```python
from build123d import *

# Parameters (mm, degrees)
F1_DEPTH  = 25.4
F2_R      = 6.2861798015
F2_R_2    = 6.4106702401
F3_DEPTH  = 12.8915009478
F5_DEPTH  = 12.8915009478
F7_DEPTH  = 69.5320936104
F10_DEPTH = 9.335500879


with BuildPart() as f1:
    # F0 (on Front) → F1 (new body)
    with BuildSketch(Plane.XZ):
        Polygon((0, 31.9150984287), (0, 0), (69.6087032557, 0), (69.6087032557, 12.8905009478), (9.334500879, 12.8905009478), (9.334500879, 31.9150984287), align=None)
    extrude(amount=F1_DEPTH)

    # F2 (on face) → F3 (cut, through all)
    with BuildSketch(Plane.XY.offset(12.8905009478)):
        with Locations((48.8061010838, -12.3570999131)):
            Circle(F2_R)
        with Locations((24.6252994984, -12.7127002925)):
            Circle(F2_R_2)
    extrude(amount=-F3_DEPTH, mode=Mode.SUBTRACT)

    # F4 (on face) → F5 (cut, through all)
    with BuildSketch(Plane.XY.offset(12.8905009478)):
        with BuildLine():
            ThreePointArc((60.931898555, 0), (69.4846296944, -13.5080407898), (58.7982981412, -25.4))
            Line((58.7982981412, -25.4), (69.6087032557, -25.4))
            Line((69.6087032557, -25.4), (69.6087032557, 0))
            Line((69.6087032557, 0), (60.931898555, 0))
        make_face()
    extrude(amount=-F5_DEPTH, mode=Mode.SUBTRACT)

    # F6 (on face) → F7 (cut, through all)
    with BuildSketch(Plane(origin=(0, 0, 0), x_dir=(0, -1, 0), z_dir=(-1, 0, 0))):
        with BuildLine():
            ThreePointArc((0, 21.0692994297), (3.4400048541, 28.1838195258), (10.4061793669, 31.9150984287))
            Line((10.4061793669, 31.9150984287), (0, 31.9150984287))
            Line((0, 31.9150984287), (0, 21.0692994297))
        make_face()
        with BuildLine():
            ThreePointArc((14.9166792368, 31.9150984287), (22.126877753, 27.9222549677), (25.4, 20.3581005335))
            Line((25.4, 20.3581005335), (25.4, 31.9150984287))
            Line((25.4, 31.9150984287), (14.9166792368, 31.9150984287))
        make_face()
    extrude(amount=-F7_DEPTH, mode=Mode.SUBTRACT)

    # F9 (on face) → F10 (cut, through all)
    with BuildSketch(Plane.YZ.offset(9.334500879)):
        with BuildLine():
            ThreePointArc((-16.6914294769, 22.3139002919), (-12.8905000165, 26.1148297523), (-9.0895705561, 22.3139002919))
            Line((-9.0895705561, 22.3139002919), (-9.0895705561, 31.6063540242))
            ThreePointArc((-9.0895705561, 31.6063540242), (-9.7437881877, 31.7781538537), (-10.4061793669, 31.9150984287))
            Line((-10.4061793669, 31.9150984287), (-14.9166792368, 31.9150984287))
            ThreePointArc((-14.9166792368, 31.9150984287), (-15.8121520335, 31.7211826291), (-16.6914294769, 31.4636053697))
            Line((-16.6914294769, 31.4636053697), (-16.6914294769, 22.3139002919))
        make_face()
        with BuildLine():
            ThreePointArc((-16.6914294769, 22.3139002919), (-12.8905000165, 18.5129708315), (-9.0895705561, 22.3139002919))
            ThreePointArc((-9.0895705561, 22.3139002919), (-12.8905000165, 26.1148297523), (-16.6914294769, 22.3139002919))
        make_face()
    extrude(amount=-F10_DEPTH, mode=Mode.SUBTRACT)


solid = f1.part
```
Model file for the job. Use its own axes, mm. A direction names the side the tool comes from. Coordinates: 2 decimals unless noted, no trailing zeros. Write each loop counter-clockwise with the first axis right and the second up, starting at its lowest first coordinate (ties: lowest second). Pieces come first, ordered by that corner, then holes. Notation, with made-up numbers: (52.5, 3.25) - (101.5, 3.25) arc R23 cw to (101.5, 12.25) - close; hole circle Ø10 at (83, -33.5). An arc over 180 degrees is marked (long way). One line per item, written item: value. Start each with the question number.
1. Slice it at D-D (y = -4.5). Write the cut outline in (x, z).
2. Slice it at B-B (x = 54). Write the cut outline in (y, z), plus the area to 3 significant figures.
3. Slice it at A-A (z = 23). Write the cut outline in (x, y).
4. Probe line 1 (X direction, y = -12.75, z = 2); line 2 (X direction, y = -15.5, z = 2); line 3 (Z direction, x = 32, y = -5.25). List the from-to ranges inside material, lowest first. Write a range as from..to.
5. Tool access for faces 1 (the flat face through (9.335, -13, 18)), 2 (the cylindrical face through (18.22, -12.43, 6.54)), 3 (the flat face through (5, -9.09, 27)): list every direction of +Z, -Z, +X, -X, +Y, -Y with a clear straight run to the whole face (end or side of a thin tool).
6. Flat gauge pins, fed straight in: pin 1 (5.5 mm diameter, centred on y = -11, z = 22.5, fed in from +X); pin 2 (1.5 mm diameter, centred on y = -18.5, z = 8, fed in from +X); pin 3 (4.5 mm diameter, centred on x = 6, z = 28.5, fed in from +Y). Where does each tip first touch, or does it go through?
7. Slice it at C-C (z = 5). Write the cut outline in (x, y).
8. Mould opens along Y. For faces 4 (the cylindrical face through (4.733, -12.974, 18.514)), 5 (the flat face through (29, -25.4, 8)), 6 (the cylindrical face through (69.5, -13.3, 6.5)), 7 (the flat face through (0, -13, 13)) say: released by +Y, released by -Y, zero draft, split by the parting line, or undercut.
Answers below:
1. outline: (0, 0) - (66.92, 0) - (66.92, 12.89) - (9.33, 12.89) - (9.33, 29.17) - (0, 29.17) - close
2. outline: (-25.4, 0) - (-15.9, 0) - (-15.9, 12.89) - (-25.4, 12.89) - close; (-8.82, 0) - (0, 0) - (0, 12.89) - (-8.82, 12.89) - close
2. area: 236 mm^2
3. outline: (0, -24.9) - (9.33, -24.9) - (9.33, -16.69) - (0, -16.69) - close; (0, -9.09) - (9.33, -9.09) - (9.33, -0.42) - (0, -0.42) - close
4. line 1: x = 0..18.21, 31.04..42.53, 55.08..69.53
4. line 2: x = 0..18.85, 30.4..43.36, 54.25..69.16
4. line 3: z = 0..12.89
5. face 1: +Z, +X, +Y, -Y
5. face 2: +Z, -Z
5. face 3: +Z, +X, -X
6. pin 1: stops at x = 9.33
6. pin 2: stops at x = 68.4
6. pin 3: stops at y = -1.91
7. outline: (0, -25.4) - (58.8, -25.4) arc R13.24 ccw to (60.93, 0) - (0, 0) - close; hole circle Ø12.82 at (24.63, -12.71); hole circle Ø12.57 at (48.81, -12.36)
8. face 4: undercut
8. face 5: released by -Y
8. face 6: split by the parting line
8. face 7: zero draft
